For this review, use the dimensioned drawing (mm, ordinates from the lowest corner) and the shaded views. A direction names the side the tool comes from. Give positions to 0.01 mm unless a question says otherwise; leave off trailing zeros. Loops run counter-clockwise (first coordinate to the right, second up) from the corner with the lowest first, then second, coordinate; pieces in that order, holes last. Notation, with made-up numbers: M 3,58 L 35,58 A19 cw 35,92 Z; hole C 44.25,36.5 d4. An arc over 180 degrees is marked long. Use CSV: the item, a comma, the result in double quotes. Start each with the question number.
1. Take a section at C-C, the plane z = 496.5. Write out the cut boundary in (x, y), and give its area (3 significant figures).
2. Take a section at A-A, the plane x = 23. Write out the cut boundary in (y, z).
3. Tool access review of the marked faces 4 and 5: name each direction out of +Z, -Z, +X, -X, +Y, -Y from which nothing blocks a thin tool from reaching the whole face with its end or side.
4. The part is to be moulded in two halves that separate along X. For the marked faces 1, 2 and 3, say which applies: pulls with the +X half, pulls with the -X half, needs draft (parallel to the pull), parting line crosses it, or undercut.
5. To check wall thickness, follow line 1 (Y direction, x = 73.5, z = 398.5). State the ranges of the line that lie inside material, in increasing order. Write a range as [from, to].
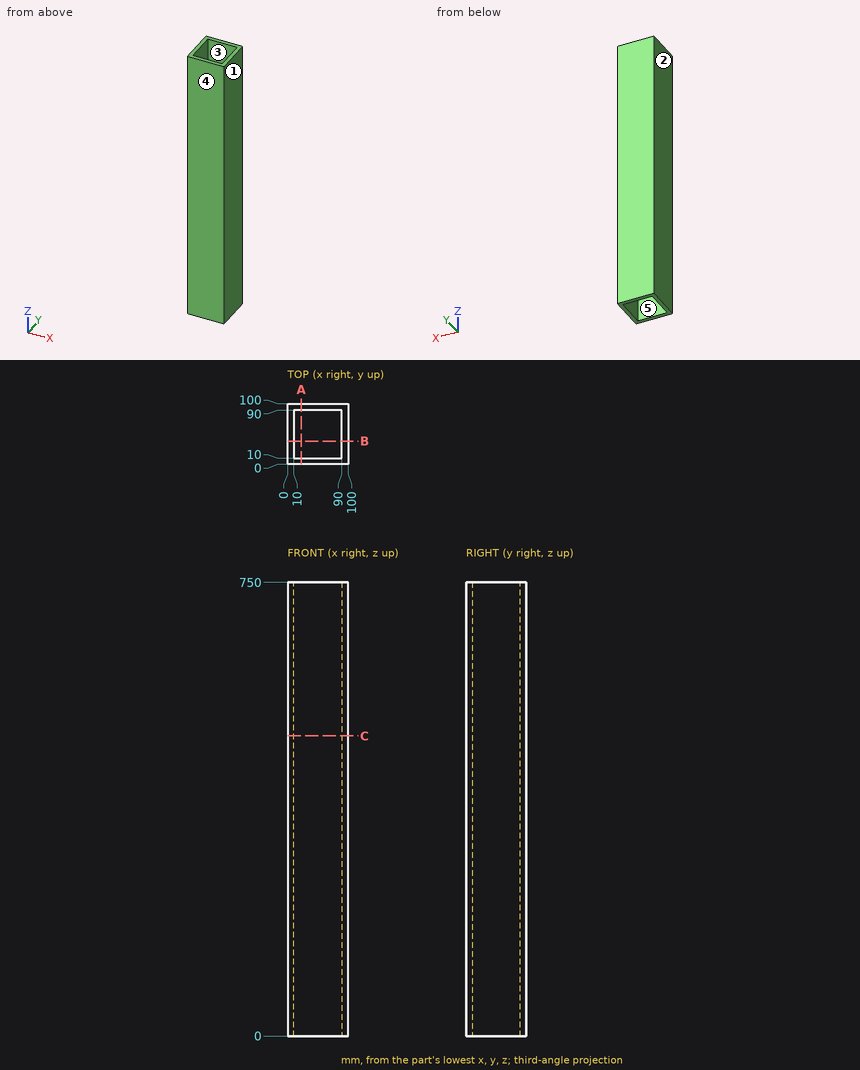
Result set:
1,outline,"M 0,0 L 100,0 L 100,100 L 0,100 Z; hole M 10,10 L 90,10 L 90,90 L 10,90 Z"
1,area,"3,600 mm2"
2,outline,"M 0,0 L 10,0 L 10,750 L 0,750 Z; M 90,0 L 100,0 L 100,750 L 90,750 Z"
3,face 4,"+Z, -Z, +X, -X, -Y"
3,face 5,"+Z, -Z"
4,face 1,"pulls with the +X half"
4,face 2,"pulls with the -X half"
4,face 3,"undercut"
5,line 1,"[0, 10], [90, 100]"
